Geometry check sheet. Reference: the model listing, model coordinates, mm. Face numbers are marked on the shaded views. A direction names the side the tool comes from. Round coordinates to 2 decimals unless told otherwise and drop trailing zeros. Write each loop counter-clockwise with the first axis right and the second up, starting at its lowest first coordinate (ties: lowest second). Pieces come first, ordered by that corner, then holes. Notation, with made-up numbers: M -20.5,11 L 32.5,11 A13 cw 32.5,30 Z; hole C 18.5,44.25 d8. An arc over 180 degrees is marked long. Answer as CSV lines item,"result". Start each with the question number.
```python
from build123d import *

# Parameters (mm, degrees)
SKETCH1_W                      = 2.5
SKETCH1_H                      = 12
BOSS_EXTRUDE1_DEPTH            = 0.5
BOSS_EXTRUDE2_DEPTH            = 9.55
F_2_5_2_5_DIAMETER_HOLE1_D     = 2.5
F_2_5_2_5_DIAMETER_HOLE1_DEPTH = 12
F_2_5_2_5_DIAMETER_HOLE1_TIP   = 0.751075774


with BuildPart() as part:
    # Sketch1 → Boss-Extrude1 (new body)
    with BuildSketch(Plane(origin=(0, 0, 0), x_dir=(1, 0, 0), z_dir=(0, 1, 0))):
        Polygon((-21.75, 31.85), (0, 31.85), (0, 76.35), (-26.25, 76.35), (-26.25, 53.35), (-26.25, 41.35), (-26.25, 31.85), align=None)
        Polygon((0, 76.35), (0, 31.85), (21.75, 31.85), (26.25, 31.85), (26.25, 76.35), align=None)
        with Locations((-27.5, 47.35)):
            Rectangle(SKETCH1_W, SKETCH1_H)
    extrude(amount=BOSS_EXTRUDE1_DEPTH)

    # Sketch1_3 → Boss-Extrude2 (add)
    with BuildSketch(Plane(origin=(0, 0, 0), x_dir=(1, 0, 0), z_dir=(0, 1, 0))):
        with BuildLine():
            Line((-28.75, 73.35), (-28.75, 53.35))
            Line((-28.75, 53.35), (-26.25, 53.35))
            Line((-26.25, 53.35), (-26.25, 79.35))
            Line((-26.25, 79.35), (-30.25, 79.35))
            ThreePointArc((-30.25, 79.35), (-33.25, 76.35), (-30.25, 73.35))
            Line((-30.25, 73.35), (-28.75, 73.35))
        make_face()
        with BuildLine():
            Line((26.25, 79.35), (26.25, 31.85))
            Line((26.25, 31.85), (21.75, 31.85))
            Line((21.75, 31.85), (21.75, 0))
            Line((21.75, 0), (28.75, 0))
            Line((28.75, 0), (28.75, 73.35))
            Line((28.75, 73.35), (30.25, 73.35))
            ThreePointArc((30.25, 73.35), (33.25, 76.35), (30.25, 79.35))
            Line((30.25, 79.35), (26.25, 79.35))
        make_face()
        Polygon((-26.25, 31.85), (-26.25, 41.35), (-28.75, 41.35), (-28.75, 0), (-21.75, 0), (-21.75, 31.85), align=None)
    extrude(amount=BOSS_EXTRUDE2_DEPTH)

    # 2.5 _2.5_ Diameter Hole1
    with Locations(Plane(origin=(0, 0, 0), x_dir=(-1, 0, 0), z_dir=(0, -1, 0))):
        with Locations((-22.85, 73.45), (22.85, 73.45), (26, 29.35), (22.85, 35.4), (-22.85, 35.4), (-26, 29.35), (-23.5, 3), (23.5, 3), (-30.25, 76.35), (30.25, 76.35)):
            Hole(F_2_5_2_5_DIAMETER_HOLE1_D / 2, depth=F_2_5_2_5_DIAMETER_HOLE1_DEPTH)
            with Locations((0, 0, -(F_2_5_2_5_DIAMETER_HOLE1_DEPTH + F_2_5_2_5_DIAMETER_HOLE1_TIP / 2))):  # 118° drill point
                Cone(0, F_2_5_2_5_DIAMETER_HOLE1_D / 2, F_2_5_2_5_DIAMETER_HOLE1_TIP, mode=Mode.SUBTRACT)


solid = part.part
```
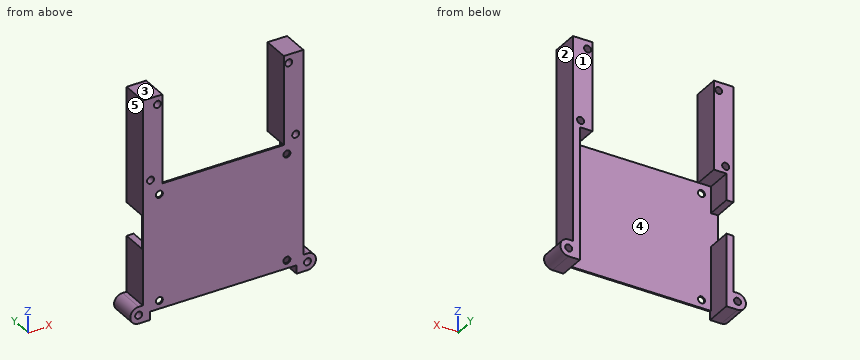
1) Section check C-C, the plane z = -25.5. Record the cut outline in (x, y).
2) Go/stop test with flat-tipped pins: pin 1 (1.3 mm diameter, centred on x = -25, y = 7, fed in from -Z); pin 2 (2 mm diameter, centred on x = -30.25, z = -76.35, fed in from +Y); pin 3 (5 mm diameter, centred on y = 5.5, z = -31.5, fed in from +X); pin 4 (4 mm diameter, centred on x = -24, z = -45.5, fed in from +Y). Record where each tip stops, or that it passes through.
3) Section check D-D, the plane x = -12. Record the cut outline in (y, z), plus the area to 4 significant figures.
4) Section check B-B, the plane z = -35.4. Record the cut outline in (x, y), plus the area to 3 significant figures.
5) Section check A-A, the plane y = 8. Give the number of separate pieces and of enclosed holes in the cut face, plus the area to 3 significant figures.
6) Mould release check, pull along X, two halves, no side actions. Record for the marked faces 3, 4 and 5: released by +X, released by -X, zero draft, split by the parting line, or undercut.
7) Scan lines: line 1 (X direction, y = 7.25, z = -29.35); line 2 (X direction, y = 0.5, z = -12); line 3 (Z direction, x = -23.5, y = 3.75). Record each from-to range of solid material in increasing order. Write a range as from..to.
8) Access from +Z, -Z, +X, -X, +Y, -Y to the whole of each face (thin tool, end or side, straight path). Record for the marked faces 1 and 2.
Results:
1,outline,"M -28.75,0 L -21.75,0 L -21.75,9.55 L -28.75,9.55 Z; M 21.75,0 L 28.75,0 L 28.75,9.55 L 21.75,9.55 Z"
2,pin 1,"stops at z = -31.85"
2,pin 2,"passes through"
2,pin 3,"stops at x = 28.75"
2,pin 4,"stops at y = 0.5"
3,outline,"M 0,-76.35 L 0.5,-76.35 L 0.5,-31.85 L 0,-31.85 Z"
3,area,"22.25 mm^2"
4,outline,"M -28.75,0 L -24.1,0 L -24.1,0.5 L -26.25,0.5 L -26.25,9.55 L -28.75,9.55 Z; M -21.6,0 L 21.6,0 L 21.6,0.5 L -21.6,0.5 Z; M 24.1,0 L 28.75,0 L 28.75,9.55 L 26.25,9.55 L 26.25,0.5 L 24.1,0.5 Z"
4,area,"71.5 mm^2"
5,separate pieces,"3"
5,enclosed holes,"6"
5,area,"670 mm^2"
6,face 3,"zero draft"
6,face 4,"undercut"
6,face 5,"released by -X"
7,line 1,"x = -28.75..-27.25, -24.75..-21.75, 21.75..24.75, 27.25..28.75"
7,line 2,"x = -28.75..-21.75, 21.75..28.75"
7,line 3,"z = -31.85..-4.25, -1.75..0"
8,face 1,"+Z, -Z, +X, -X, +Y"
8,face 2,"+Z, +X, +Y, -Y"
